Autodesk Inventor part; units mm, degrees
ref_plane "YZ Plane" through (0, 0, 0) normal (1, 0, 0) x (0, 1, 0)
ref_plane "XZ Plane" through (0, 0, 0) normal (0, 1, 0) x (-1, 0, 0)
ref_plane "XY Plane" through (0, 0, 0) normal (0, 0, 1) x (1, 0, 0)
sketch "Sketch1" plane through (0, 0, 0) normal (0, 0, 1) x (1, 0, 0)
  line L0 (1.4722, 2.55) -> (2.9445, 0)
  line L1 (2.9445, 0) -> (1.4722, -2.55)
  line L2 (1.4722, -2.55) -> (-1.4722, -2.55)
  line L3 (-1.4722, -2.55) -> (-2.9445, 0)
  line L4 (-2.9445, 0) -> (-1.4722, 2.55)
  line L5 (-1.4722, 2.55) -> (1.4722, 2.55)
  point P0 (0, 0)
  dimension "d0" = 5.1
extrude "Extrusion1" add sketch "Sketch1" along normal blind 0.4
sketch "Sketch2" plane through (0, 0, 0.4) normal (0, 0, 1) x (1, 0, 0)
  circle A0 centre (0, 0) radius 2.4
  dimension "d3" = 4.8
extrude "Extrusion2" add sketch "Sketch2" along normal blind 8.6
sketch "Sketch3" plane through (0, 0, 9) normal (0, 0, 1) x (1, 0, 0)
  circle A0 centre (0, 0) radius 2.4
  circle A1 centre (0, 0) radius 1.5
  dimension "d6" = 3
extrude "Extrusion3" cut sketch "Sketch3" against normal blind 10 contours A1
chamfer "Chamfer1" distance 0.3 angle 45 1 edges at (-1.5, 0, 9)
thread "Thread1"
properties part number "Вытяжная заклепка_Р-Ш-М3-Ум" material "Сталь низкоуглеродистая"
Design review of the part built by this model. Coordinates are the model's own, in mm. A direction names the side the tool comes from. Coordinates: 2 decimals unless noted, no trailing zeros. Order: outer loops, then holes, each group sorted by start corner. A loop starts at its lowest first (then second) coordinate and runs counter-clockwise, first axis right, second up.
Item 1: Take a section at B-B, the plane y = 2.15. Write out the cut boundary in (x, z), then the cut area to 3 significant figures.
Item 2: Take a section at A-A, the plane x = 0. Write out the cut boundary in (y, z), then the cut area to 3 significant figures.
Item 3: The part is to be moulded in two halves that separate along Y. For faces 3 (the flat face through (1.3, 1.2, 0)), 4 (the flat face through (2.219, -1.257, 0.197)), 5 (the flat face through (-2.219, 1.257, 0.197)), 6 (the cylindrical face through (-1.5, 0.07, 4.41)), say which applies: pulls with the +Y half, pulls with the -Y half, needs draft (parallel to the pull), parting line crosses it, or undercut.
Item 4: Take a section at D-D, the plane x = -2.6. Write out the cut boundary in (y, z).
Item 5: For faces 1 (the flat face through (-2.2, -1.29, 0.2)), 2 (the cylindrical face through (1.29, -2.024, 4.64)), list the 3-axis set-ups (+Z, -Z, +X, -X, +Y, -Y) from which the entire face can be reached by the end or side of a thin tool; tool diameter is ignored.
Item 6: For pin 1 Ø1 at (y, z) = (0, 6.5) entering from +X; pin 2 Ø2 at (x, z) = (-0.5, 4.5) entering from -Y; pin 3 Ø2.5 at (x, y) = (0, 0) entering from +Z; pin 4 Ø1.5 at (x, z) = (-1.5, 8) entering from -Y, all flat-tipped, find the tip position at first contact; note any pin that passes through.
Item 7: Take a section at C-C, the plane z = 4.75. Write out the cut boundary in (x, y).
Item 8: For line 1 (Y direction, x = 0, z = 2.25); line 2 (Z direction, x = -2.7, y = -0.2); line 3 (X direction, y = 0.3, z = 3), list the stretches that pass through material, from the lowest coordinate up.
The answers:
1. outline: (-1.7, 0) - (1.7, 0) - (1.7, 0.4) - (1.07, 0.4) - (1.07, 9) - (-1.07, 9) - (-1.07, 0.4) - (-1.7, 0.4) - close
1. area: 19.7 mm2
2. outline: (-2.55, 0) - (-1.5, 0) - (-1.5, 8.7) - (-1.8, 9) - (-2.4, 9) - (-2.4, 0.4) - (-2.55, 0.4) - close; (1.5, 0) - (2.55, 0) - (2.55, 0.4) - (2.4, 0.4) - (2.4, 9) - (1.8, 9) - (1.5, 8.7) - close
2. area: 16.2 mm2
3. face 3: needs draft
3. face 4: pulls with the -Y half
3. face 5: pulls with the +Y half
3. face 6: undercut
4. outline: (-0.6, 0) - (0.6, 0) - (0.6, 0.4) - (-0.6, 0.4) - close
5. face 1: +Z, -Z, -X, -Y
5. face 2: +Z
6. pin 1: stops at x = 2.4
6. pin 2: stops at y = -2.4
6. pin 3: passes through
6. pin 4: stops at y = -2.28
7. outline: circle Ø4.8 at (0, 0); hole circle Ø3 at (0, 0)
8. line 1: y = -2.4 to -1.5, 1.5 to 2.4
8. line 2: z = 0 to 0.4
8. line 3: x = -2.38 to -1.47, 1.47 to 2.38
